Design review of the part built by this model. Coordinates are the model's own, in mm. Face numbers are marked on the shaded views. A direction names the side the tool comes from. Give positions to 0.01 mm unless a question says otherwise; leave off trailing zeros. Loops run counter-clockwise (first coordinate to the right, second up) from the corner with the lowest first, then second, coordinate; pieces in that order, holes last. Notation, with made-up numbers: (-13.75, -25.75) -> (36.25, -25.75) arc R23 ccw to (36.25, -16.75) -> close; hole circle Ø10 at (65.5, 17). An arc over 180 degrees is marked (long way). Use a Markdown table: item, result. Add a question column.
1. For the marked faces 1, 2 and 3, list the 3-axis set-ups (+Z, -Z, +X, -X, +Y, -Y) from which the entire face can be reached by the end or side of a thin tool; tool diameter is ignored.
2. Add section A-A (y = 72). State the section outline as (x, z) points (3 decimals), and give its area (3 significant figures).
3. Add section C-C (z = -29). State the section outline as (x, y) points.
4. To check wall thickness, follow line 1 (Y direction, x = 25, z = 34.5) (3 decimals); line 2 (Z direction, x = 37.5, y = 72); line 3 (Z direction, x = 6.5, y = 75). State the ranges of each line that lie inside material, in increasing order.
5. For pin 1 Ø2.5 at (x, y) = (41, 78) entering from -Z; pin 2 Ø5 at (x, y) = (20.5, 30.5) entering from -Z; pin 3 Ø2.5 at (x, z) = (27, 22) entering from -Y, all flat-tipped, find the tip position at first contact; note any pin that passes through.
6. Add section B-B (z = 33.5). State the section outline as (x, y) points (3 decimals), and give its area (3 significant figures).
7. Add section D-D (z = -17). State the section outline as (x, y) points.
```python
from build123d import *

# Parameters (mm, degrees)
BOSS_EXTRUDE1_DEPTH = 88.9
BOSS_EXTRUDE2_DEPTH = 44.45
CUT_EXTRUDE1_DEPTH  = 12.7
CUT_EXTRUDE2_DEPTH  = 44.45


with BuildPart() as part:
    # Sketch2 → Boss-Extrude1 (new body)
    with BuildSketch(Plane(origin=(0, 0, 0), x_dir=(1, 0, 0), z_dir=(0, 1, 0))):
        with BuildLine():
            Line((0, 0), (0, 50.8))
            Line((0, 50.8), (15.226765087, 50.8))
            ThreePointArc((15.226765087, 50.8), (28.988508692, 40.599003798), (36.890166373, 25.4))
            Line((36.890166373, 25.4), (44.45, 25.4))
            Line((44.45, 25.4), (44.45, -44.45))
            Line((44.45, -44.45), (0, -44.45))
            Line((0, -44.45), (0, 0))
        make_face()
    extrude(amount=BOSS_EXTRUDE1_DEPTH)

    # Sketch3 → Boss-Extrude2 (add)
    with BuildSketch(Plane(origin=(44.45, 0, 0), x_dir=(0, 0, -1), z_dir=(1, 0, 0))):
        with BuildLine():
            Line((25.4, 66.675), (25.4, 22.225))
            ThreePointArc((25.4, 22.225), (47.625, 44.45), (25.4, 66.675))
        make_face()
    extrude(amount=-BOSS_EXTRUDE2_DEPTH)

    # Sketch4 → Cut-Extrude1 (cut)
    with BuildSketch(Plane(origin=(44.45, 0, 0), x_dir=(0, 0, -1), z_dir=(1, 0, 0))):
        with BuildLine():
            ThreePointArc((34.925, 44.45), (32.135192091, 51.185192091), (25.4, 53.975))
            Line((25.4, 53.975), (25.4, 34.925))
            ThreePointArc((25.4, 34.925), (32.135192091, 37.714807909), (34.925, 44.45))
        make_face()
        with BuildLine():
            Line((25.4, 34.925), (25.4, 53.975))
            ThreePointArc((25.4, 53.975), (15.875, 44.45), (25.4, 34.925))
        make_face()
    extrude(amount=-CUT_EXTRUDE1_DEPTH, mode=Mode.SUBTRACT)

    # Sketch5 → Cut-Extrude2 (cut)
    with BuildSketch(Plane(origin=(44.45, 0, 0), x_dir=(0, 0, -1), z_dir=(1, 0, 0))):
        Polygon((0, 88.9), (-44.45, 88.9), (-44.45, 60.325), (-23.8125, 60.325), (-23.8125, 55.5625), (-19.05, 55.5625), (-19.05, 60.325), (0, 60.325), align=None)
        Polygon((-23.8125, 28.575), (-44.45, 28.575), (-44.45, 0), (0, 0), (0, 28.575), (-19.05, 28.575), (-19.05, 33.3375), (-23.8125, 33.3375), align=None)
    extrude(amount=-CUT_EXTRUDE2_DEPTH, mode=Mode.SUBTRACT)


solid = part.part
```
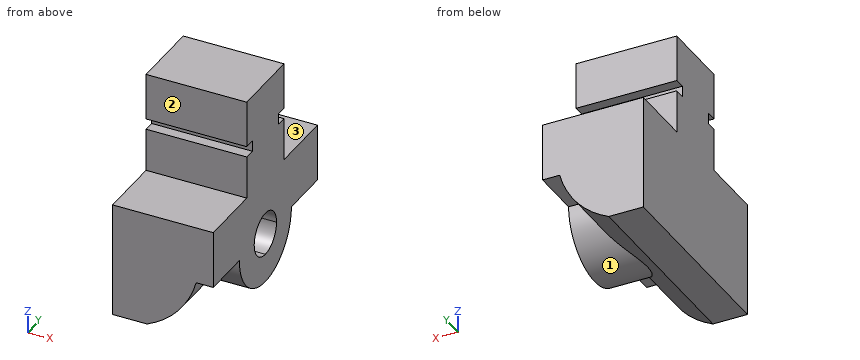
Taken from the geometry:
| question | item | result |
|---|---|---|
| 1 | face 1 | -Z, +X |
| 1 | face 2 | +Z, +X, -X, -Y |
| 1 | face 3 | +Z, +X, -X, +Y |
| 2 | outline | (0, -50.8) -> (15.227, -50.8) arc R38.1 ccw to (36.89, -25.4) -> (44.45, -25.4) -> (44.45, 0) -> (0, 0) -> close |
| 2 | area | 1,880 mm^2 |
| 3 | outline | (0, 0) -> (35.77, 0) -> (35.77, 22.52) -> (44.45, 22.52) -> (44.45, 35.63) -> (31.75, 35.63) -> (31.75, 53.27) -> (44.45, 53.27) -> (44.45, 66.38) -> (35.77, 66.38) -> (35.77, 88.9) -> (0, 88.9) -> close |
| 4 | line 1 | y = 28.575 to 60.325 |
| 4 | line 2 | z = -25.4 to 0 |
| 4 | line 3 | z = -50.8 to 0 |
| 5 | pin 1 | stops at z = -25.4 |
| 5 | pin 2 | stops at z = -49.45 |
| 5 | pin 3 | stops at y = 33.34 |
| 6 | outline | (0, 28.575) -> (44.45, 28.575) -> (44.45, 60.325) -> (0, 60.325) -> close |
| 6 | area | 1,410 mm^2 |
| 7 | outline | (0, 0) -> (44.45, 0) -> (44.45, 39.96) -> (31.75, 39.96) -> (31.75, 48.94) -> (44.45, 48.94) -> (44.45, 88.9) -> (0, 88.9) -> close |
